Part model, mm, in its own coordinate system. Face numbers are marked on the shaded views. Coordinates: 2 decimals unless noted, no trailing zeros. Write each loop counter-clockwise with the first axis right and the second up, starting at its lowest first coordinate (ties: lowest second). Pieces come first, ordered by that corner, then holes. Notation, with made-up numbers: M 10,-11.5 L 63,-11.5 A23 ccw 63,21.5 Z; hole C 34,-26 d4. An arc over 180 degrees is marked long. Use a Markdown table: item, result. Add a question column.
Q1. Pin check, flat tips, straight feed: pin 1 Ø8 at (x, z) = (13, 11) entering from -Y; pin 2 Ø3 at (x, z) = (-15, 4) entering from +Y; pin 3 Ø2 at (y, z) = (-4.5, 16.5) entering from -X. Stop position of each tip, or through.
Q2. Mould opens along Y. For the marked faces 1 and 2 say: released by +Y, released by -Y, zero draft, split by the parting line, or undercut.
Q3. Slice it at A-A on y = -12.5. Write the cut outline in (x, z), then the cut area to 3 significant figures.
Q4. Wall check: L1, parallel to Y at x = -25, z = 14.5; L2, parallel to X at y = -25.5, z = 17.75. Give the ranges that are in metal, low to high. Write a range as from..to.
Q5. Slice it at B-B on x = -3.5. Write the cut outline in (y, z).
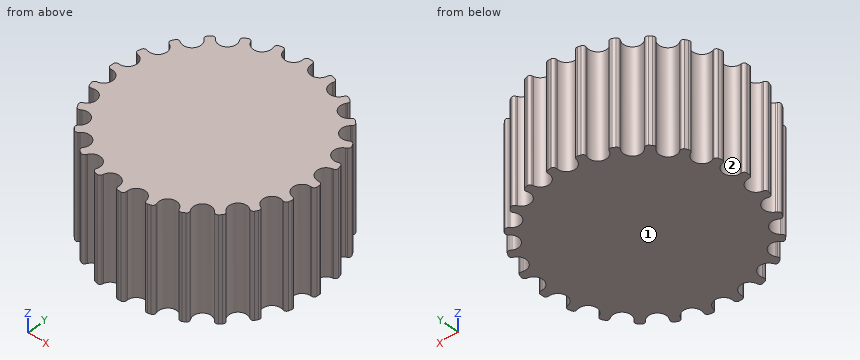
from build123d import *

# Parameters (mm, degrees)
SKETCH2_R         = 29.875
EXTRUDE1_DEPTH    = 30
EXTRUDE2_DEPTH    = 30
CIRPATTERN1_COUNT = 24


with BuildPart() as part:
    # Sketch2 → Extrude1 (new body)
    with BuildSketch(Plane.XY):
        Circle(SKETCH2_R)
    extrude(amount=EXTRUDE1_DEPTH)

    # Sketch1 → Extrude2 (cut)
    with BuildSketch(Plane.XY):
        with BuildLine():
            Line((-1.206491179, 29.085066823), (-1.202957444, 28.680140914))
            ThreePointArc((-1.202957444, 28.680140914), (-3.437407272, 26.109700424), (-6.260999022, 28.014237108))
            Line((-6.260999022, 28.014237108), (-6.362388233, 28.406280098))
            ThreePointArc((-6.362388233, 28.406280098), (-6.719671358, 28.881877013), (-7.308355692, 28.967284341))
            ThreePointArc((-7.308355692, 28.967284341), (-3.899469993, 29.619415234), (-0.437955362, 29.871789704))
            ThreePointArc((-0.437955362, 29.871789704), (-0.98447572, 29.636929843), (-1.206491179, 29.085066823))
        make_face()
    extrude2 = extrude(amount=EXTRUDE2_DEPTH, mode=Mode.SUBTRACT)

    # CirPattern1: Extrude2 ×24 about axis
    cirpattern1_axis = Axis((0, 0, 0), (0, 0, 1))
    for i in range(1, CIRPATTERN1_COUNT):
        add(extrude2.rotate(cirpattern1_axis, i * 360 / CIRPATTERN1_COUNT), mode=Mode.SUBTRACT)


solid = part.part
Recorded:
| question | item | result |
|---|---|---|
| 1 | pin 1 | y = -26.19 |
| 1 | pin 2 | y = 26.19 |
| 1 | pin 3 | x = -26.75 |
| 2 | face 1 | zero draft |
| 2 | face 2 | undercut |
| 3 | outline | M -24.58,0 L 24.58,0 L 24.58,30 L -24.58,30 Z |
| 3 | area | 1,470 mm² |
| 4 | L1 | -15.7..-12.98, -9.14..9.14, 12.98..15.7 |
| 4 | L2 | -15.5..-13.33, -8.79..8.79, 13.33..15.5 |
| 5 | outline | M -26.1,0 L 26.1,0 L 26.1,30 L -26.1,30 Z |
